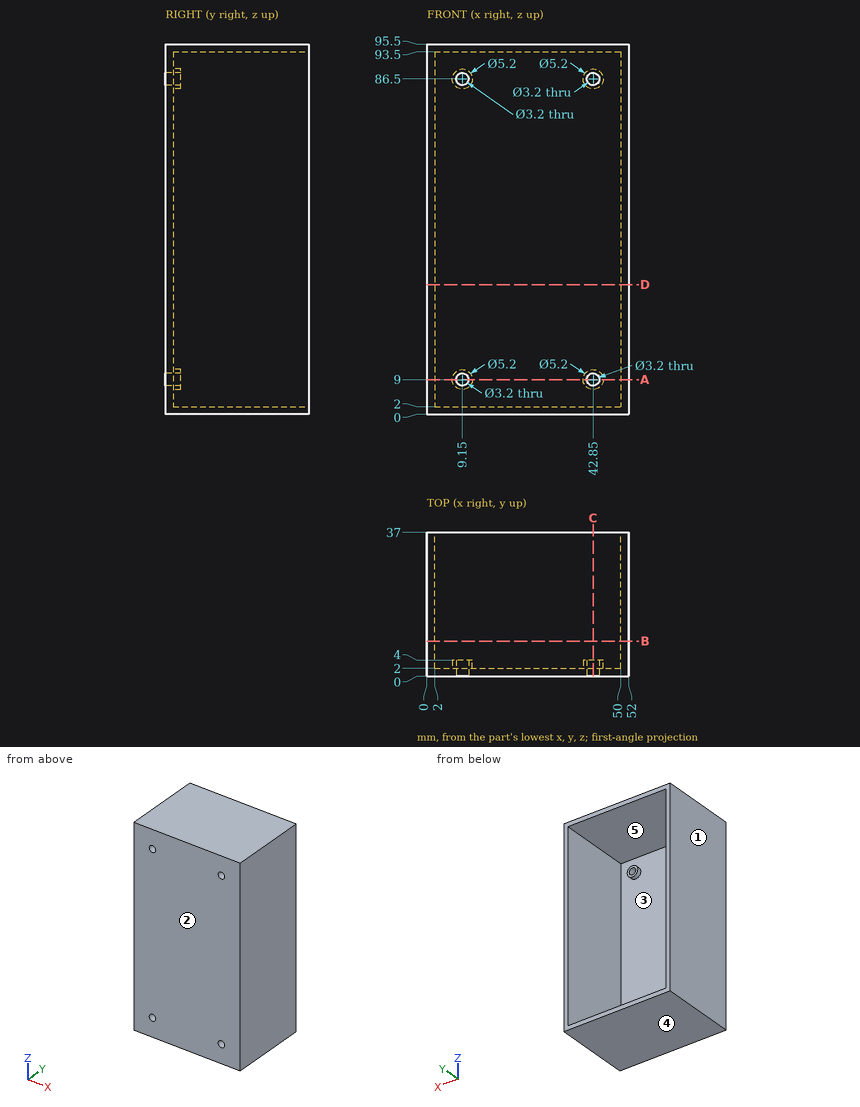
For this review, use the dimensioned drawing (mm, ordinates from the lowest corner) and the shaded views. A direction names the side the tool comes from. Round coordinates to 2 decimals unless told otherwise and drop trailing zeros. Write each loop counter-clockwise with the first axis right and the second up, starting at its lowest first coordinate (ties: lowest second). Pieces come first, ordered by that corner, then holes. Notation, with made-up numbers: M -30.75,-3.5 L 11.25,-3.5 A23 cw 11.25,31.5 Z; hole C 5,38.5 d3. An arc over 180 degrees is marked long. Use CSV: the item, a comma, the result in double quotes. Start each with the question number.
(1) We need section B-B, the plane y = 9. State the section outline as (x, z) points, then the cut area to 3 significant figures.
(2) We need section D-D, the plane z = 33.5. State the section outline as (x, y) points.
(3) Clearance check with flat-ended pins moving along their axes: P1, Ø4, axis at x = 43.5, z = 87, coming from the +Y side; P2, Ø4, axis at x = 36, z = 66.5, coming from the +Y side. State where each tip first meets the part, or that it passes through.
(4) We need section A-A, the plane z = 9. State the section outline as (x, y) points, then the cut area to 3 significant figures.
(5) Tool access review of the marked faces 4 and 5: name each direction out of +Z, -Z, +X, -X, +Y, -Y from which nothing blocks a thin tool from reaching the whole face with its end or side.
(6) The part is to be moulded in two halves that separate along X. For the marked faces 1, 2 and 3, say which applies: +X half, -X half, draft (parallel to the pull), parting line (faces both ways), or undercut.
(7) For line 1 along X through (y, z) = (2.7, 86.5); line 2 along Z through (x, y) = (42.85, 2.7); line 3 along X through (y, z) = (1, 9), list the stretches that pass through material, from the lowest coordinate up.
(8) We need section C-C, the plane x = 42.85. State the section outline as (y, z) points, then the cut area to 3 significant figures.
Findings:
1,outline,"M 0,0 L 52,0 L 52,95.5 L 0,95.5 Z; hole M 2,2 L 50,2 L 50,93.5 L 2,93.5 Z"
1,area,"574 mm^2"
2,outline,"M 0,0 L 52,0 L 52,37 L 50,37 L 50,2 L 2,2 L 2,37 L 0,37 Z"
3,P1,"y = 4"
3,P2,"y = 2"
4,outline,"M 0,0 L 7.55,0 L 7.55,4 L 6.55,4 L 6.55,2 L 2,2 L 2,37 L 0,37 Z; M 10.75,0 L 41.25,0 L 41.25,4 L 40.25,4 L 40.25,2 L 11.75,2 L 11.75,4 L 10.75,4 Z; M 44.45,0 L 52,0 L 52,37 L 50,37 L 50,2 L 45.45,2 L 45.45,4 L 44.45,4 Z"
4,area,"239 mm^2"
5,face 4,"-Z, +X, -X, +Y, -Y"
5,face 5,"+Y"
6,face 1,"-X half"
6,face 2,"draft"
6,face 3,"undercut"
7,line 1,"0 to 2, 6.55 to 7.55, 10.75 to 11.75, 40.25 to 41.25, 44.45 to 45.45, 50 to 52"
7,line 2,"0 to 2, 6.4 to 7.4, 10.6 to 11.6, 83.9 to 84.9, 88.1 to 89.1, 93.5 to 95.5"
7,line 3,"0 to 7.55, 10.75 to 41.25, 44.45 to 52"
8,outline,"M 0,0 L 37,0 L 37,2 L 2,2 L 2,6.4 L 4,6.4 L 4,7.4 L 0,7.4 Z; M 0,10.6 L 4,10.6 L 4,11.6 L 2,11.6 L 2,83.9 L 4,83.9 L 4,84.9 L 0,84.9 Z; M 0,88.1 L 4,88.1 L 4,89.1 L 2,89.1 L 2,93.5 L 37,93.5 L 37,95.5 L 0,95.5 Z"
8,area,"326 mm^2"
